Check sheet for the modelled part. Datum: model origin and axes. Units: mm. A direction names the side the tool comes from. Coordinates: 2 decimals unless noted, no trailing zeros. Loops run counter-clockwise (first coordinate to the right, second up) from the corner with the lowest first, then second, coordinate; pieces in that order, holes last. Notation, with made-up numbers: M -9,-33 L 17,-33 A21 ccw 17,-24 Z; hole C -34.5,-10.75 d4. An arc over 180 degrees is marked long. Answer in a Markdown table with one row per item. Add a question column.
Autodesk Inventor part; units mm, degrees
ref_plane "YZ Plane" through (0, 0, 0) normal (1, 0, 0) x (0, 1, 0)
ref_plane "XZ Plane" through (0, 0, 0) normal (0, 1, 0) x (-1, 0, 0)
ref_plane "XY Plane" through (0, 0, 0) normal (0, 0, 1) x (1, 0, 0)
sketch "Sketch1" plane through (0, 0, 0) normal (0, 1, 0) x (-1, 0, 0)
  line L0 (-17.5, 17.5) -> (17.5, -17.5) construction
  line L1 (17.5, 17.5) -> (-17.5, -17.5) construction
  circle A0 centre (17.5, 17.5) radius 1.25
  circle A1 centre (-17.5, 17.5) radius 1.25
  circle A2 centre (17.5, -17.5) radius 1.25
  circle A3 centre (-17.5, -17.5) radius 1.25
  line L2 (-20, 20) -> (20, 20)
  line L3 (20, 20) -> (20, -20)
  line L4 (20, -20) -> (-20, -20)
  line L5 (-20, -20) -> (-20, 20)
  line L6 (-20, 20) -> (20, -20) construction
  line L7 (20, 20) -> (-20, -20) construction
  point P0 (0, 0)
  dimension "d0" = 35
  dimension "d1" = 35
  dimension "d2" = 2.5
  dimension "d3" = 2.5
  dimension "d4" = 2.5
  dimension "d5" = 2.5
  dimension "d6" = 40
  dimension "d7" = 40
extrude "Extrusion2" add sketch "Sketch1" along normal blind 3
sketch "Sketch2" plane through (0, 3, 0) normal (0, 1, 0) x (1, 0, 0)
  line L0 (20, -15) -> (-20, -15)
  line L1 (-20, -15) -> (-20, 15)
  line L2 (-20, 15) -> (20, 15)
  line L3 (20, 15) -> (20, -15)
  line L4 (20, -15) -> (-20, 15) construction
  line L5 (-20, -15) -> (20, 15) construction
  line L6 (-13.5, 10) -> (13.5, 10)
  line L7 (13.5, 10) -> (13.5, 20)
  line L8 (13.5, 20) -> (-13.5, 20)
  line L9 (-13.5, 20) -> (-13.5, 10)
  line L10 (-13.5, 10) -> (13.5, 20) construction
  line L11 (13.5, 10) -> (-13.5, 20) construction
  line L12 (-13.5, -10) -> (13.5, -10)
  line L13 (13.5, -10) -> (13.5, -20)
  line L14 (13.5, -20) -> (-13.5, -20)
  line L15 (-13.5, -20) -> (-13.5, -10)
  line L16 (-13.5, -10) -> (13.5, -20) construction
  line L17 (13.5, -10) -> (-13.5, -20) construction
  point P0 (0, 0)
  point P1 (0, 15)
  point P2 (0, -15)
  point P3 (13.5, -15)
  point P4 (-13.5, -15)
  point P5 (-13.5, 15)
  point P6 (13.5, 15)
  dimension "d12" = 40
  dimension "d13" = 30
  dimension "d27" = 27
  dimension "d28" = 10
  dimension "d29" = 27
  dimension "d30" = 10
extrude "Extrusion3" add sketch "Sketch2" along normal blind 15
sketch "Sketch4" plane through (-20, 0, -20) normal (-1, 0, 0) x (0, 0, 1)
  line L0 (0, 0) -> (40, 0)
  line L1 (40, 0) -> (40, 3)
  line L2 (35, 3) -> (40, 3)
  line L3 (35, 3) -> (35, 18)
  line L4 (5, 18) -> (35, 18)
  line L5 (5, 3) -> (5, 18)
  line L6 (0, 3) -> (5, 3)
  line L7 (0, 0) -> (0, 3)
  line L8 (33.5, -17) -> (6.5, -17)
  line L9 (6.5, -17) -> (6.5, 17)
  line L10 (6.5, 17) -> (33.5, 17)
  line L11 (33.5, 17) -> (33.5, -17)
  line L12 (33.5, -17) -> (6.5, 17) construction
  line L13 (6.5, -17) -> (33.5, 17) construction
  line L14 (5, 18) -> (6.5, 18)
  line L15 (6.5, 18) -> (6.5, 0)
  line L16 (6.5, 0) -> (5, 0)
  line L17 (5, 0) -> (5, 18)
  line L18 (5, 18) -> (35, 18)
  line L19 (35, 18) -> (33.5, 18)
  line L20 (33.5, 18) -> (33.5, 0)
  line L21 (33.5, 0) -> (35, 0)
  line L22 (35, 0) -> (35, 18)
  line L23 (6.5, 17) -> (5, 17)
  line L24 (33.5, 17) -> (35, 17)
  point P0 (20, 0)
  dimension "d20" = 27
  dimension "d21" = 34
extrude "Extrusion5" cut sketch "Sketch4" against normal blind 31 contours L17 L5 L23 L9 L0 | L9 L10 L11 L0 | L11 L24 L3 L22 L0
chamfer "Chamfer2" distance 2 angle 45 2 edges at (-4.5, 0, -15) (-4.5, 0, 15)
chamfer "Chamfer3" distance 4 angle 45 6 edges at (20, 10.5, -15) (13.5, 10.5, -20) (-13.5, 10.5, -20) (-13.5, 10.5, 20) (13.5, 10.5, 20) (20, 10.5, 15)
properties part number "obudowa_gps_bt" material "ABS Plastic"
Q1. Cross-section at C-C (y = 1.5). Record the cut outline in (x, z).
Q2. Thickness scan on L1, parallel to Z at x = -9.5, y = 9.75; L2, parallel to Z at x = -12.5, y = 9.5; L3, parallel to Y at x = -7, z = -14. Record the ranges inside material, lowest first.
Q3. Mould release check, pull along Z, two halves, no side actions. Record for faces 1 (the face through (11.5, 10.6, -18)), 2 (the face through (16, 3, 17)), 3 (the face through (-1, 9, -15)): released by +Z, released by -Z, zero draft, split by the parting line, or undercut.
Q4. Cross-section at B-B (x = -17.5). Record the cut outline in (y, z), plus the area to 3 significant figures.
Q5. Access from +Z, -Z, +X, -X, +Y, -Y to the whole of each face (thin tool, end or side, straight path). Record for faces 4 (the face through (-5, 17, 0)), 5 (the face through (13.5, 10.4, 15.5)), 6 (the face through (-16, 3, -17)), 7 (the face through (16, 3, -17)), 8 (the face through (-16, 3, 18)).
Q6. Cross-section at A-A (z = -17.5). Record the cut outline in (x, y).
Q7. Cross-section at D-D (x = 17.5). Record the cut outline in (y, z), plus the area to 3 significant figures.
Q8. Go/stop test with flat-tipped pins: pin 1 (0.8 mm diameter, centred on y = 7.5, z = 15.5, fed in from +X); pin 2 (0.5 mm diameter, centred on y = 8, z = -15.5, fed in from -X); pin 3 (1 mm diameter, centred on x = 7, z = 16, fed in from -Y). Record where each tip stops, or that it passes through.
Answer key:
| question | item | result |
|---|---|---|
| 1 | outline | M -20,-20 L 20,-20 L 20,20 L -20,20 L -20,15.5 L 11,15.5 L 11,-15.5 L -20,-15.5 Z; hole C -17.5,-17.5 d2.5; hole C -17.5,17.5 d2.5; hole C 17.5,-17.5 d2.5; hole C 17.5,17.5 d2.5 |
| 2 | L1 | -20 to -15, 15 to 20 |
| 2 | L2 | -17 to -15, 15 to 17 |
| 2 | L3 | 17 to 18 |
| 3 | face 1 | released by -Z |
| 3 | face 2 | zero draft |
| 3 | face 3 | undercut |
| 4 | outline | M 0,-20 L 3,-20 L 3,-18.75 L 0,-18.75 Z; M 0,18.75 L 3,18.75 L 3,20 L 0,20 Z; M 0.75,-16.25 L 3,-16.25 L 3,-15 L 2,-15 Z; M 0.75,16.25 L 2,15 L 3,15 L 3,16.25 Z; M 17,-15 L 18,-15 L 18,15 L 17,15 Z |
| 4 | area | 41.6 mm^2 |
| 5 | face 4 | -X, -Y |
| 5 | face 5 | +Z, +X, +Y |
| 5 | face 6 | -Z, -X, +Y |
| 5 | face 7 | -Z, +X, +Y |
| 5 | face 8 | +Z, -X, +Y |
| 6 | outline | M -20,0 L -18.75,0 L -18.75,3 L -20,3 Z; M -16.25,0 L 16.25,0 L 16.25,3 L 12,3 L 12,18 L -12,18 L -12,3 L -16.25,3 Z; M 18.75,0 L 20,0 L 20,3 L 18.75,3 Z |
| 7 | outline | M 0,-20 L 3,-20 L 3,-18.75 L 0,-18.75 Z; M 0,-16.25 L 3,-16.25 L 3,-13.5 L 18,-13.5 L 18,13.5 L 3,13.5 L 3,16.25 L 0,16.25 Z; M 0,18.75 L 3,18.75 L 3,20 L 0,20 Z |
| 7 | area | 510 mm^2 |
| 8 | pin 1 | x = 13.5 |
| 8 | pin 2 | x = -13.5 |
| 8 | pin 3 | y = 0.5 |
